Answer from the drawing. Dimensions are ordinates in mm from the lowest x, y and z of the part. A direction names the side the tool comes from. Coordinates: 2 decimals unless noted, no trailing zeros. Write each loop counter-clockwise with the first axis right and the second up, starting at its lowest first coordinate (ties: lowest second). Pieces come first, ordered by that corner, then holes.
(1) The part is cut by section A-A on x = 22.78. Determine the outline of the cut face in (y, z).
(2) The part is cut by section B-B on z = 8.4. Determine the outline of the cut face in (x, y), plus the area to 3 significant figures.
(3) Given P1, Ø1.5, axis at x = 7, z = 8, coming from the -Y side, flat-ended and moving along its own axis, determine where the tip first touches the part or whether it passes through.
(4) Straight lines are drawn through the part: line 1 (X direction, y = 8.65, z = 3.4); line 2 (X direction, y = 8.5, z = 4); line 3 (Y direction, x = 1.75, z = 10.25). For each, find the intervals that lie inside material, in ascending order.
(5) Which of the six approach directions +Z, -Z, +X, -X, +Y, -Y give full straight-line access (tool end or side, diameter ignored) to the marked faces 1 and 2?
(6) The part is cut by section D-D on z = 11. Determine the outline of the cut face in (x, y), plus the area to 3 significant figures.
(7) The part is cut by section C-C on x = 16. Determine the outline of the cut face in (y, z).
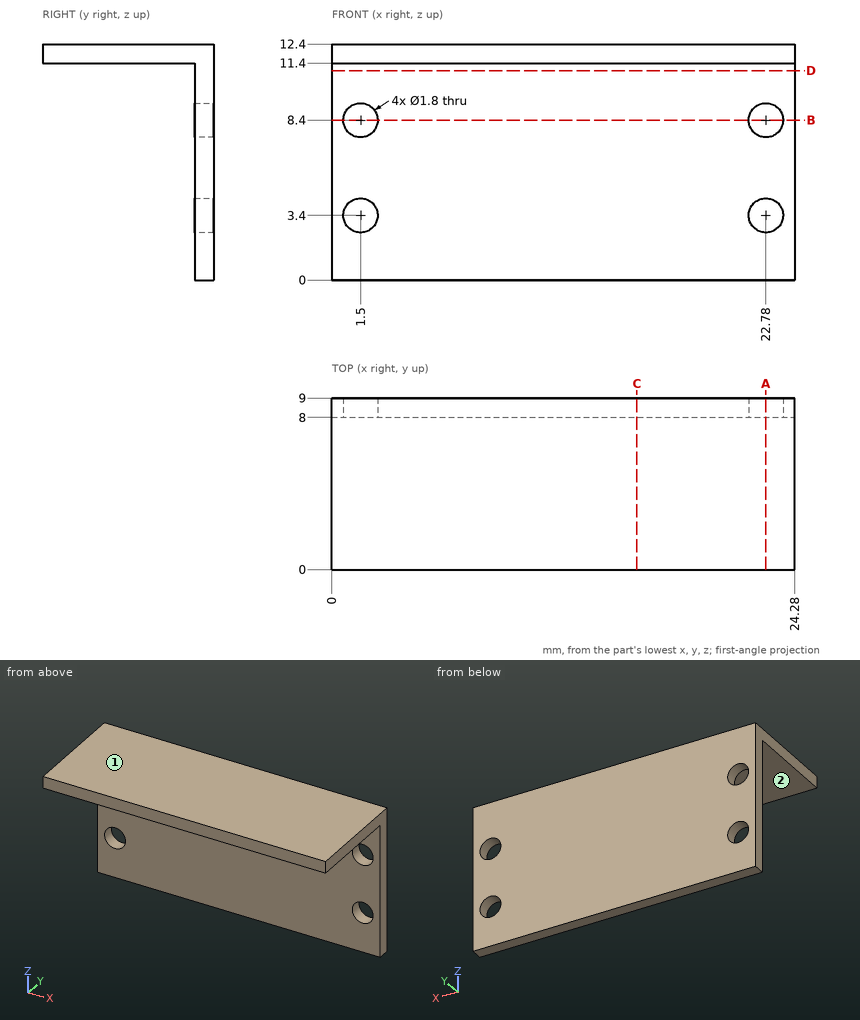
Model answer:
1. outline: (0, 11.4) - (8, 11.4) - (8, 9.3) - (9, 9.3) - (9, 12.4) - (0, 12.4) - close; (8, 0) - (9, 0) - (9, 2.5) - (8, 2.5) - close; (8, 4.3) - (9, 4.3) - (9, 7.5) - (8, 7.5) - close
2. outline: (0, 8) - (0.6, 8) - (0.6, 9) - (0, 9) - close; (2.4, 8) - (21.88, 8) - (21.88, 9) - (2.4, 9) - close; (23.68, 8) - (24.28, 8) - (24.28, 9) - (23.68, 9) - close
2. area: 20.7 mm2
3. P1: stops at y = 8
4. line 1: x = 0 to 0.6, 2.4 to 21.88, 23.68 to 24.28
4. line 2: x = 0 to 0.83, 2.17 to 22.11, 23.45 to 24.28
4. line 3: y = 8 to 9
5. face 1: +Z, +X, -X, +Y, -Y
5. face 2: -Z, +X, -X, -Y
6. outline: (0, 8) - (24.28, 8) - (24.28, 9) - (0, 9) - close
6. area: 24.3 mm2
7. outline: (0, 11.4) - (8, 11.4) - (8, 0) - (9, 0) - (9, 12.4) - (0, 12.4) - close
